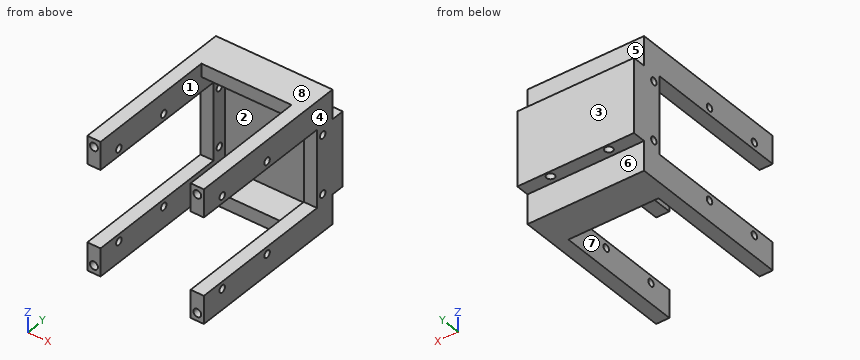
Autodesk Inventor part; units mm, degrees
ref_plane "YZ Plane" through (0, 0, 0) normal (1, 0, 0) x (0, 1, 0)
ref_plane "XZ Plane" through (0, 0, 0) normal (0, 1, 0) x (-1, 0, 0)
ref_plane "XY Plane" through (0, 0, 0) normal (0, 0, 1) x (1, 0, 0)
sketch "스케치1" plane through (0, 0, 0) normal (0, 1, 0) x (-1, 0, 0)
  line L0 (22, -14) -> (-22, -14)
  line L1 (-22, -14) -> (-22, 14)
  line L2 (-22, 14) -> (22, 14)
  line L3 (22, 14) -> (22, -14)
  point P0 (0, 0)
  dimension "d0" = 44
  dimension "d1" = 22
  dimension "d2" = 28
  dimension "d3" = 14
extrude "돌출1" add sketch "스케치1" along normal blind 5
sketch "스케치2" plane through (-22, 0, 14) normal (0, 0, 1) x (1, 0, 0)
  circle A0 centre (33, 3) radius 1.5
  circle A1 centre (11, 3) radius 1.5
  line L0 (44, 0) -> (0, 0)
  line L1 (22, 0) -> (22, 5)
  line L2 (44, 5) -> (0, 5)
  dimension "d6" = 3
  dimension "d7" = 3
  dimension "d8" = 3
  dimension "d9" = 3
  dimension "d10" = 22
  dimension "d11" = 11
extrude "돌출2" cut sketch "스케치2" against normal blind 60
sketch "스케치3" plane through (0, 0, 0) normal (0, -1, 0) x (1, 0, 0)
  line L0 (-17, 14.5) -> (17, 14.5)
  line L1 (17, 14.5) -> (17, -14.5)
  line L2 (17, -14.5) -> (-17, -14.5)
  line L3 (-17, -14.5) -> (-17, 14.5)
  line L4 (22, -14) -> (-22, -14)
  line L5 (22, 25.1) -> (-22, 25.1)
  line L6 (-22, 25.1) -> (-22, -25.1)
  line L7 (-22, -25.1) -> (22, -25.1)
  line L8 (22, -25.1) -> (22, 25.1)
  point P0 (0, 0)
  dimension "d17" = 34
  dimension "d18" = 17
  dimension "d20" = 29
  dimension "d21" = 14.5
  dimension "d22" = 10.6
  dimension "d23" = 10.6
  dimension "d24" = 5
  dimension "d25" = 5
extrude "돌출3" add sketch "스케치3" along normal blind 2
sketch "스케치4" plane through (0, -2, 0) normal (0, -1, 0) x (1, 0, 0)
  line L0 (-22, 25.1) -> (-22, -25.1)
  line L1 (-22, -25.1) -> (22, -25.1)
  line L2 (-22, 25.1) -> (22, 25.1)
  line L3 (22, 25.1) -> (22, -25.1)
  line L4 (22, -25.1) -> (-22, -25.1)
  line L5 (-22, -25.1) -> (-22, 25.1)
  line L6 (-17, 20.1) -> (17, 20.1)
  line L7 (17, 20.1) -> (17, -20.1)
  line L8 (17, -20.1) -> (-17, -20.1)
  line L9 (-17, -20.1) -> (-17, 20.1)
  point P0 (0, 0)
  dimension "d28" = 5
  dimension "d29" = 5
  dimension "d30" = 5
  dimension "d31" = 5
extrude "돌출4" add sketch "스케치4" along normal blind 5.58
sketch "스케치5" plane through (22, 5, 14) normal (1, 0, 0) x (0, 0, -1)
  circle A0 centre (25, -9.8) radius 1.35
  circle A1 centre (3, -9.8) radius 1.35
  line L0 (39.1, -5) -> (28, -5)
  line L1 (0, -5) -> (-11.1, -5)
  point P0 (14, -5)
  dimension "d34" = 2.7
  dimension "d35" = 2.7
  dimension "d36" = 4.8
  dimension "d37" = 4.8
  dimension "d38" = 22
  dimension "d39" = 11
extrude "돌출5" cut sketch "스케치5" against normal blind 90
sketch "스케치6" plane through (0, -7.58, 0) normal (0, -1, 0) x (1, 0, 0)
  line L0 (22, -25.1) -> (-22, -25.1)
  line L1 (-22, -25.1) -> (-22, -20.1)
  line L2 (-22, -20.1) -> (22, -20.1)
  line L3 (22, -20.1) -> (22, -25.1)
  line L4 (22, 25.1) -> (-22, 25.1)
  line L5 (-22, 25.1) -> (-22, 20.1)
  line L6 (-22, 20.1) -> (22, 20.1)
  line L7 (22, 20.1) -> (22, 25.1)
  point P0 (0, 0)
  dimension "d42" = 5
  dimension "d43" = 5
extrude "돌출6" add sketch "스케치6" along normal blind 6
sketch "스케치7" plane through (0, -7.58, 0) normal (0, -1, 0) x (1, 0, 0)
  line L0 (22, -20.1) -> (-22, -20.1)
  line L1 (17, 20.1) -> (17, -20.1)
  line L2 (22, -20.1) -> (17, -20.1)
  line L3 (17, -20.1) -> (17, -14.6)
  line L4 (17, -14.6) -> (22, -14.6)
  line L5 (22, -14.6) -> (22, -20.1)
  line L6 (22, 14) -> (22, 25.1)
  line L7 (22, 20.1) -> (17, 20.1)
  line L8 (17, 20.1) -> (17, 14.6)
  line L9 (17, 14.6) -> (22, 14.6)
  line L10 (22, 14.6) -> (22, 20.1)
  line L11 (-22, -14) -> (-22, 14)
  line L12 (-17, -20.1) -> (-22, -20.1)
  line L13 (-22, -20.1) -> (-22, -14.6)
  line L14 (-22, -14.6) -> (-17, -14.6)
  line L15 (-17, -14.6) -> (-17, -20.1)
  line L16 (-17, 20.1) -> (-22, 20.1)
  line L17 (-22, 20.1) -> (-22, 14.6)
  line L18 (-22, 14.6) -> (-17, 14.6)
  line L19 (-17, 14.6) -> (-17, 20.1)
  line L20 (22, 20.1) -> (17, 20.1)
  point P0 (0, 0)
  dimension "d46" = 5.5
  dimension "d47" = 5.5
  dimension "d48" = 5.5
  dimension "d49" = 5.5
  dimension "d50" = 0
extrude "돌출7" add sketch "스케치7" along normal blind 55.52
sketch "스케치8" plane through (0, -13.58, 0) normal (0, -1, 0) x (1, 0, 0)
  line L0 (-22, -20.1) -> (-22, -25.1)
  line L1 (-17, -20.1) -> (-22, -20.1)
  line L2 (-22, -25.1) -> (-17, -25.1)
  line L3 (-17, -25.1) -> (-17, -20.1)
  line L4 (-17, -20.1) -> (-22, -20.1)
  line L5 (-22, -20.1) -> (-22, -25.1)
  line L6 (-17, -20.1) -> (17, -20.1)
  line L7 (22, -25.1) -> (22, -20.1)
  line L8 (17, -20.1) -> (22, -20.1)
  line L9 (22, -20.1) -> (22, -25.1)
  line L10 (22, -25.1) -> (17, -25.1)
  line L11 (17, -25.1) -> (17, -20.1)
  line L12 (17, -20.1) -> (17, 20.1)
  line L13 (22, 20.1) -> (22, 25.1)
  line L14 (17, 20.1) -> (22, 20.1)
  line L15 (22, 20.1) -> (22, 25.1)
  line L16 (22, 25.1) -> (17, 25.1)
  line L17 (17, 25.1) -> (17, 20.1)
  line L18 (-22, 25.1) -> (-22, 20.1)
  line L19 (22, 25.1) -> (-22, 25.1)
  line L20 (-22, 20.1) -> (-17, 20.1)
  line L21 (-17, 20.1) -> (-17, 25.1)
  line L22 (-17, 25.1) -> (-22, 25.1)
  line L23 (-22, 25.1) -> (-22, 20.1)
  point P0 (0, 0)
extrude "돌출8" add sketch "스케치8" along normal blind 49.52
sketch "스케치9" plane through (-22, 5, -14) normal (-1, 0, 0) x (0, 0, 1)
  circle A0 centre (31.3, -59.1) radius 1.35
  circle A1 centre (-3.3, -59.1) radius 1.35
  line L0 (-0.6, -68.1) -> (-11.1, -68.1)
  line L1 (39.1, -68.1) -> (28.6, -68.1)
  line L2 (39.1, -5) -> (39.1, -68.1)
  line L3 (-11.1, -5) -> (-11.1, -68.1)
  circle A2 centre (31.3, -37.1) radius 1.35
  circle A3 centre (-3.3, -37.1) radius 1.35
  point P0 (14, -5)
  dimension "d55" = 9
  dimension "d56" = 9
  dimension "d57" = 2.7
  dimension "d58" = 2.7
  dimension "d59" = 7.8
  dimension "d60" = 7.8
  dimension "d61" = 2.7
  dimension "d62" = 2.7
  dimension "d63" = 22
  dimension "d64" = 22
extrude "돌출9" cut sketch "스케치9" against normal blind 49.52
sketch "스케치10" plane through (0, -63.1, 0) normal (0, -1, 0) x (1, 0, 0)
  circle A0 centre (19.5, 22.1) radius 1.5
  line L0 (22, 14.6) -> (22, 25.1)
  line L1 (22, 25.1) -> (17, 25.1)
  line L2 (0, 0) -> (14.9637, 0)
  line L3 (0, 0) -> (0, 14.6)
  circle A1 centre (19.5, -22.1) radius 1.5
  circle A2 centre (-19.5, 22.1) radius 1.5
  circle A3 centre (-19.5, -22.1) radius 1.5
  dimension "d67" = 2.5
  dimension "d68" = 3
  dimension "d69" = 3
extrude "돌출10" cut sketch "스케치10" against normal blind 10
properties part number "elbow"
CAD build for the part. Positions are in the model's coordinates, mm. Face numbers are marked on the shaded views. A direction names the side the tool comes from. Round coordinates to 2 decimals unless told otherwise and drop trailing zeros. Loops run counter-clockwise (first coordinate to the right, second up) from the corner with the lowest first, then second, coordinate; pieces in that order, holes last. Notation, with made-up numbers: M 59.25,-18 L 76.25,-18 A22 ccw 76.25,8 Z; hole C 24.25,27.5 d9. An arc over 180 degrees is marked long. One line per question, with ' | ' between items. Start each with the question number.
Item 1: Cut at A-A, the plane y = 3. Write the cut outline in (x, z).
Item 2: Two-plate mould, pull along X, no slides. Class the marked faces 1, 2, 3 and 4: pulls with the +X half, pulls with the -X half, needs draft (parallel to the pull), parting line crosses it, or undercut.
Item 3: Wall check: line 1 (Y direction, x = 18.7, z = 17.3); line 2 (X direction, y = -46, z = 16); line 3 (Y direction, x = -20, z = -11). Give the ranges that are in metal, low to high.
Item 4: Cut at D-D, the plane y = -4.8. Write the cut outline in (x, z), plus the area to 3 significant figures.
Item 5: Cut at B-B, the plane z = 11. Write the cut outline in (x, y).
Item 6: Which spindle directions (+Z, -Z, +X, -X, +Y, -Y) get a long thin tool onto all of the face, cutting with end or side? Do the marked faces 5, 6, 7 and 8. Say none if no direction does.
Item 7: Pin check, flat tips, straight feed: pin 1 Ø3.5 at (y, z) = (-4.8, -11) entering from -X; pin 2 Ø10 at (x, z) = (12, 20) entering from +Y; pin 3 Ø1.5 at (x, z) = (20, -22) entering from -Y; pin 4 Ø1.5 at (x, z) = (-20.5, 0) entering from -Y. Stop position of each tip, or through.
Item 8: Cut at C-C, the plane x = 19.5. Write the cut outline in (y, z).
Responses:
1) outline: M -22,-14 L -12.5,-14 L -12.5,14 L -22,14 Z; M -9.5,-14 L 9.5,-14 L 9.5,14 L -9.5,14 Z; M 12.5,-14 L 22,-14 L 22,14 L 12.5,14 Z
2) face 1: undercut | face 2: undercut | face 3: needs draft | face 4: pulls with the +X half
3) line 1: y = -63.1 to -55.45, -52.75 to -33.45, -30.75 to 0 | line 2: x = -22 to -17, 17 to 22 | line 3: y = -7.58 to -6.15, -3.45 to 5
4) outline: M -22,-25.1 L 22,-25.1 L 22,-12.35 L 17,-12.35 L 17,-20.1 L -17,-20.1 L -17,-12.35 L -22,-12.35 Z; M -22,-9.65 L -17,-9.65 L -17,9.65 L -22,9.65 Z; M -22,12.35 L -17,12.35 L -17,20.1 L 17,20.1 L 17,12.35 L 22,12.35 L 22,25.1 L -22,25.1 Z; M 17,-9.65 L 22,-9.65 L 22,9.65 L 17,9.65 Z | area: 788 mm²
5) outline: M -22,-7.58 L -17,-7.58 L -17,-6.15 L -22,-6.15 Z; M -22,-3.45 L -17,-3.45 L -17,-2 L 17,-2 L 17,-3.45 L 22,-3.45 L 22,5 L -22,5 Z; M 17,-7.58 L 22,-7.58 L 22,-6.15 L 17,-6.15 Z; hole C -11,3 d3; hole C 11,3 d3
6) face 5: +Z, +X, -X, +Y | face 6: -Z, +X, -X, +Y | face 7: -Y | face 8: +Z, +X, -X, +Y, -Y
7) pin 1: stops at x = -22 | pin 2: stops at y = 0 | pin 3: stops at y = -53.1 | pin 4: stops at y = -7.58
8) outline: M -63.1,-25.1 L 0,-25.1 L 0,-14 L 5,-14 L 5,14 L 0,14 L 0,25.1 L -63.1,25.1 L -63.1,23.6 L -53.1,23.6 L -53.1,20.6 L -63.1,20.6 L -63.1,14.6 L -7.58,14.6 L -7.58,-14.6 L -63.1,-14.6 L -63.1,-20.6 L -53.1,-20.6 L -53.1,-23.6 L -63.1,-23.6 Z; hole C -54.1,-17.3 d2.7; hole C -54.1,17.3 d2.7; hole C -32.1,-17.3 d2.7; hole C -32.1,17.3 d2.7; hole C -4.8,-11 d2.7; hole C -4.8,11 d2.7
